from build123d import *

# Parameters (mm, degrees)
SKETCH_W     = 200
SKETCH_H     = 130
SKETCH_R     = 35
SKETCH_R_2   = 1.5625
PAD_DEPTH    = 12
SKETCH001_R  = 40
POCKET_DEPTH = 10
FILLET_R     = 3


with BuildPart() as part:
    # Sketch → Pad (new body)
    with BuildSketch(Plane.XY):
        with Locations((100, 65)):
            Rectangle(SKETCH_W, SKETCH_H)
        with Locations((100, 65)):
            Circle(SKETCH_R, mode=Mode.SUBTRACT)
        with Locations((45, 115)):
            Circle(SKETCH_R_2, mode=Mode.SUBTRACT)
        with Locations((45, 15)):
            Circle(SKETCH_R_2, mode=Mode.SUBTRACT)
        with Locations((155, 115)):
            Circle(SKETCH_R_2, mode=Mode.SUBTRACT)
        with Locations((155, 15)):
            Circle(SKETCH_R_2, mode=Mode.SUBTRACT)
        with Locations((185, 30)):
            Circle(SKETCH_R_2, mode=Mode.SUBTRACT)
        with Locations((135.353085, 100.338453)):
            Circle(SKETCH_R_2, mode=Mode.SUBTRACT)
        with Locations((64.627773, 29.642413)):
            Circle(SKETCH_R_2, mode=Mode.SUBTRACT)
        with Locations((64.64463, 100.35537)):
            Circle(SKETCH_R_2, mode=Mode.SUBTRACT)
        with Locations((135.352442, 29.63292)):
            Circle(SKETCH_R_2, mode=Mode.SUBTRACT)
        with Locations((175, 20)):
            Circle(SKETCH_R_2, mode=Mode.SUBTRACT)
        with Locations((175, 40)):
            Circle(SKETCH_R_2, mode=Mode.SUBTRACT)
        with Locations((185, 50)):
            Circle(SKETCH_R_2, mode=Mode.SUBTRACT)
        with Locations((175, 90)):
            Circle(SKETCH_R_2, mode=Mode.SUBTRACT)
        with Locations((175, 110)):
            Circle(SKETCH_R_2, mode=Mode.SUBTRACT)
        with Locations((185, 80)):
            Circle(SKETCH_R_2, mode=Mode.SUBTRACT)
        with Locations((185, 100)):
            Circle(SKETCH_R_2, mode=Mode.SUBTRACT)
        with Locations((15, 30)):
            Circle(SKETCH_R_2, mode=Mode.SUBTRACT)
        with Locations((25, 20)):
            Circle(SKETCH_R_2, mode=Mode.SUBTRACT)
        with Locations((25, 40)):
            Circle(SKETCH_R_2, mode=Mode.SUBTRACT)
        with Locations((15, 50)):
            Circle(SKETCH_R_2, mode=Mode.SUBTRACT)
        with Locations((25, 90)):
            Circle(SKETCH_R_2, mode=Mode.SUBTRACT)
        with Locations((25, 110)):
            Circle(SKETCH_R_2, mode=Mode.SUBTRACT)
        with Locations((15, 80)):
            Circle(SKETCH_R_2, mode=Mode.SUBTRACT)
        with Locations((15, 100)):
            Circle(SKETCH_R_2, mode=Mode.SUBTRACT)
    extrude(amount=PAD_DEPTH)

    # Sketch001 (on Face31 of Pad) → Pocket (cut)
    with BuildSketch(Plane.XY.offset(12)):
        with Locations((100, 65)):
            Circle(SKETCH001_R)
    extrude(amount=-POCKET_DEPTH, mode=Mode.SUBTRACT)

    # Fillet
    fillet_edges = [part.edges().sort_by_distance(p)[0] for p in [
        (200, 0, 6),
        (200, 130, 6),
        (0, 0, 6),
        (0, 130, 6),
    ]]
    fillet(fillet_edges, radius=FILLET_R)


solid = part.part
Source: CAD feature listing. Evaluate the final solid. Frame: model axes, mm. A direction names the side the tool comes from. Coordinates: 2 decimals unless noted, no trailing zeros. Loops run counter-clockwise (first coordinate to the right, second up) from the corner with the lowest first, then second, coordinate; pieces in that order, holes last. Notation, with made-up numbers: (-12.75, 52.25) - (45.25, 52.25) arc R34 ccw to (45.25, 84.25) - close; hole circle Ø11 at (59.5, 9.5). An arc over 180 degrees is marked (long way). One line per question, with ' | ' between items.
1) Section B-B, the plane y = 95. Return loops of the section in (x, z), then the cut area to 3 significant figures.
Report:
outline: (0, 0) - (81.97, 0) - (81.97, 2) - (73.54, 2) - (73.54, 12) - (0, 12) - close; (118.03, 0) - (200, 0) - (200, 12) - (126.46, 12) - (126.46, 2) - (118.03, 2) - close | area: 1,800 mm²
2) First-contact query: P1, Ø3.5, axis at x = 135.35, y = 100.34, coming from the +Z side; P2, Ø1.9, axis at x = 15, y = 100, coming from the -Z side. Flat tips, straight axial feed; report the tip coordinate or a pass-through.
Report:
P1: stops at z = 12 | P2: passes through
3) Set-up query: faces 5 (the face through (0, 64, 6)), 6 (the face through (138.153, 77.015, 7.07)). Return all of +Z, -Z, +X, -X, +Y, -Y with unobstructed straight access to the full face (end or side cutting, diameter ignored); none if empty.
Report:
face 5: +Z, -Z, -X, +Y, -Y | face 6: +Z
4) Pull-direction query (Y, two-part tool) for faces 1 (the face through (99, 0, 6)), 2 (the face through (99.8, 29.6, 2)), 3 (the face through (76, 95, 0)), 4 (the face through (99, 130, 6)); classes: released by +Y, released by -Y, zero draft, split by the parting line, or undercut.
Report:
face 1: released by -Y | face 2: undercut | face 3: zero draft | face 4: released by +Y
5) Section A-A, the plane x = 100. Return loops of the section in (y, z), then the cut area to 3 significant figures.
Report:
outline: (0, 0) - (30, 0) - (30, 2) - (25, 2) - (25, 12) - (0, 12) - close; (100, 0) - (130, 0) - (130, 12) - (105, 12) - (105, 2) - (100, 2) - close | area: 620 mm²
6) Section C-C, the plane z = 7.5. Give the number of separate pieces and of enclosed holes in the cut face, then the cut area to 3 significant figures.
Report:
separate pieces: 1 | enclosed holes: 25 | area: 20,800 mm²
7) Line query: line 1 along Y through (x, z) = (175, 7); line 2 along Y through (x, z) = (185, 2.5); line 3 along X through (y, z) = (99, 8.5). Output: solid intervals per line, ascending.
Report:
line 1: y = 0 to 18.44, 21.56 to 38.44, 41.56 to 88.44, 91.56 to 108.44, 111.56 to 130 | line 2: y = 0 to 28.44, 31.56 to 48.44, 51.56 to 78.44, 81.56 to 98.44, 101.56 to 130 | line 3: x = 0 to 13.8, 16.2 to 63.87, 65.42 to 78.93, 121.07 to 134.55, 136.16 to 183.8, 186.2 to 200
